Source: CAD feature listing. Evaluate the final solid. Frame: model axes, mm. A direction names the side the tool comes from. Round coordinates to 2 decimals unless told otherwise and drop trailing zeros. Order: outer loops, then holes, each group sorted by start corner. A loop starts at its lowest first (then second) coordinate and runs counter-clockwise, first axis right, second up. Notation, with made-up numbers: (6.25, -36) -> (40.25, -36) arc R19 cw to (40.25, -17) -> close; hole circle Ø9 at (86, 17.5). An arc over 180 degrees is marked (long way). Use a Markdown table: item, result. Add a question column.
Autodesk Inventor part; units mm, degrees
ref_plane "YZ Plane" through (0, 0, 0) normal (1, 0, 0) x (0, 1, 0)
ref_plane "XZ Plane" through (0, 0, 0) normal (0, 1, 0) x (-1, 0, 0)
ref_plane "XY Plane" through (0, 0, 0) normal (0, 0, 1) x (1, 0, 0)
sketch "Sketch1" plane through (0, 0, 0) normal (0, 1, 0) x (-1, 0, 0)
  line L0 (-21, 21) -> (21, 21)
  line L1 (21, 21) -> (21, -21)
  line L2 (21, -21) -> (-21, -21)
  line L3 (-21, -21) -> (-21, 21)
  line L4 (-21, 21) -> (21, -21) construction
  line L5 (21, 21) -> (-21, -21) construction
  point P0 (0, 0)
  dimension "d0" = 42
  dimension "d1" = 42
extrude "Extrusion1" add sketch "Sketch1" along normal blind 101.6
sketch "Sketch2" plane through (0, 101.6, 0) normal (0, 1, 0) x (1, 0, 0)
  line L0 (21, 21) -> (-21, 21)
  line L1 (0, 21) -> (0, 18)
  line L2 (0, 18) -> (-18, 18)
  line L3 (-18, 18) -> (18, 18)
  line L4 (18, 18) -> (18, 14)
  line L5 (18, 14) -> (-18, 14)
  line L6 (-18, 14) -> (-18, 18)
  line L7 (21, -21) -> (21, 21)
  point P0 (0, 0)
  dimension "d4" = 3
  dimension "d5" = 18
  dimension "d6" = 36
  dimension "d7" = 4
extrude "Extrusion2" cut sketch "Sketch2" against normal through all
sketch "Sketch3" plane through (21, 0, -21) normal (0, 0, -1) x (-1, 0, 0)
  line L0 (0, 101.6) -> (42, 101.6)
  line L1 (21, 101.6) -> (21, 0)
  line L2 (21, 50.8) -> (39, 50.8)
  line L3 (39, 101.6) -> (39, 0)
  circle A0 centre (21, 50.8) radius 2.125
  dimension "d10" = 4.25
extrude "Extrusion3" cut sketch "Sketch3" against normal blind 3 contours A0 L2 L1 | L1 A0 | L2 A0 L1
pattern_linear "Rectangular Pattern1" count 2 spacing 12 along (-1, 0, 0) count 4 spacing 12 along (0, 1, 0) of "Extrusion3"
pattern_linear "Rectangular Pattern2" count 4 spacing 12 along (0, 1, 0) count 2 spacing 12 along (1, 0, 0) of "Extrusion3"
sketch "Sketch4" plane through (-21, 0, -21) normal (-1, 0, 0) x (0, 0, 1)
  line L0 (42, 0) -> (42, 101.6)
  line L1 (7, 101.6) -> (7, 0)
  line L2 (7, 72.8791) -> (9, 72.8791)
  line L3 (0, 101.6) -> (42, 101.6)
  line L4 (19.3629, 101.6) -> (19.3629, 91.6)
  line L5 (21, 91.6) -> (28.5, 91.6)
  line L6 (28.5, 91.6) -> (28.5, 76.6)
  line L7 (28.5, 76.6) -> (13.5, 76.6)
  line L8 (13.5, 76.6) -> (13.5, 91.6)
  line L9 (13.5, 91.6) -> (21, 91.6)
  point P0 (21, 0)
  dimension "d25" = 2
  dimension "d26" = 10
  dimension "d27" = 91.6
  dimension "d30" = 7.5
  dimension "d31" = 15
  dimension "d32" = 15
  dimension "d33" = 15
extrude "Extrusion4" cut sketch "Sketch4" against normal through all
sketch "Sketch5" plane through (21, 0, -21) normal (0, 0, -1) x (-1, 0, 0)
  point P0 (21, 0)
sketch "Sketch6" plane through (0, 0, 0) normal (0, -1, 0) x (1, 0, 0)
  line L0 (-18, -14) -> (18, -14)
  line L1 (18, -14) -> (18, -18)
  line L2 (18, -18) -> (-18, -18)
  line L3 (-18, -18) -> (-18, -14)
  line L4 (-18, -14) -> (18, -18) construction
  line L5 (18, -14) -> (-18, -18) construction
  point P0 (0, 0)
  point P1 (0, -16)
extrude "Extrusion5" add sketch "Sketch6" against normal blind 45
sketch "Sketch7" plane through (0, 101.6, 0) normal (0, 1, 0) x (1, 0, 0)
  line L0 (-18, 18) -> (-18, -18)
  line L1 (-21, -21) -> (21, -21)
  line L2 (-18, -18) -> (18, -18)
  line L3 (18, 18) -> (18, 14)
  line L4 (18, -18) -> (18, 18)
  line L5 (18, 18) -> (-18, 18)
  point P0 (0, 0)
  dimension "d38" = 36
  dimension "d39" = 36
extrude "Extrusion6" cut sketch "Sketch7" against normal through all
sketch "Sketch8" plane through (21, 0, -21) normal (0, 0, -1) x (-1, 0, 0)
  line L0 (-0.2731, 24.5) -> (42.2731, 24.5)
  line L1 (42.2731, 24.5) -> (42.2731, -24.5)
  line L2 (42.2731, -24.5) -> (-0.2731, -24.5)
  line L3 (-0.2731, -24.5) -> (-0.2731, 24.5)
  line L4 (-0.2731, 24.5) -> (42.2731, -24.5) construction
  line L5 (42.2731, 24.5) -> (-0.2731, -24.5) construction
  point P0 (21, 0)
  dimension "d42" = 49
extrude "Extrusion7" cut sketch "Sketch8" against normal through all
sketch "Sketch9" plane through (21, 101.6, -21) normal (0, 0, -1) x (-1, 0, 0)
  circle A0 centre (33, -26.8) radius 2.125
  circle A1 centre (33, -38.8) radius 2.125
  line L0 (33, -26.8) -> (33, -38.8)
  line L1 (33, -32.8) -> (42, -32.8)
  line L2 (42, -77.1) -> (42, 0)
  line L3 (42, -32.8) -> (0, -32.8)
  line L4 (0, -32.8) -> (0, 0)
  line L5 (0, 0) -> (42, 0)
  line L6 (42, 0) -> (42, -32.8)
  circle A2 centre (21, -26.8) radius 2.125
  line L7 (21, -32.8) -> (21, -26.8)
  line L8 (42, -77.1) -> (39, -77.1)
  line L9 (0, -77.1) -> (42, -77.1)
  point P0 (21, -101.6)
  dimension "d45" = 42
  dimension "d46" = 32.8
properties part number "CraneArmBase"
1) Reachability of faces 1 (the flat face through (-20, 76.6, 0)), 2 (the cylindrical face through (-11.723, 52.907, -19.521)), 3 (the flat face through (4, 64, -18)) from +Z, -Z, +X, -X, +Y, -Y: full face, straight path, thin tool, end or side. Return the list, or none.
2) Section D-D on x = -6.5. Output: boundary loops of the cut face in (y, z).
3) Section A-A on x = -12. Output: boundary loops of the cut face in (y, z) (3 decimals).
4) Line query: probe 1 along Y at (x, z) = (-12, -19.8) (3 decimals); probe 2 along X at (y, z) = (62.8, -19) (3 decimals); probe 3 along Z at (x, y) = (9, 64.5). Output: solid intervals per line, ascending. Write a range as from..to.
5) First-contact query: pin 1 Ø6 at (y, z) = (83, 3.5) entering from +X; pin 2 Ø7 at (x, y) = (12, 74.8) entering from -Z; pin 3 Ø2.5 at (x, y) = (12, 62.8) entering from -Z. Flat tips, straight axial feed; report the tip coordinate or a pass-through.
6) Section C-C on z = -4. Output: boundary loops of the cut face in (x, y).
7) Section B-B on y = 86.8. Output: boundary loops of the cut face in (x, z) (3 decimals), then the cut area to 3 significant figures.
8) Draft query along Z for faces 4 (the cylindrical face through (0.277, 64.907, -19.521)), 5 (the flat face through (-5, 63, -21)), 6 (the flat face through (0, 63, 21)), 7 (the flat face through (-20, 84, 7.5)). Return one class per face: pulls with the +Z half, pulls with the -Z half, needs draft (parallel to the pull), parting line crosses it, or undercut.
Conclusion:
| question | item | result |
|---|---|---|
| 1 | face 1 | +X, -X |
| 1 | face 2 | -Z |
| 1 | face 3 | +Y, -Y |
| 2 | outline | (24.5, -21) -> (101.6, -21) -> (101.6, -18) -> (24.5, -18) -> close; (24.5, 18) -> (101.6, 18) -> (101.6, 21) -> (24.5, 21) -> close |
| 3 | outline | (24.5, -21) -> (48.675, -21) -> (48.675, -18) -> (24.5, -18) -> close; (24.5, 18) -> (101.6, 18) -> (101.6, 21) -> (24.5, 21) -> close; (52.925, -21) -> (60.675, -21) -> (60.675, -18) -> (52.925, -18) -> close; (64.925, -21) -> (72.675, -21) -> (72.675, -18) -> (64.925, -18) -> close; (76.925, -21) -> (84.675, -21) -> (84.675, -18) -> (76.925, -18) -> close; (88.925, -21) -> (101.6, -21) -> (101.6, -18) -> (88.925, -18) -> close |
| 4 | probe 1 | y = 24.5..48.675, 52.925..60.675, 64.925..72.675, 76.925..84.675, 88.925..101.6 |
| 4 | probe 2 | x = -21..-14.125, -9.875..-2.125, 2.125..9.875, 14.125..21 |
| 4 | probe 3 | z = -21..-18, 18..21 |
| 5 | pin 1 | passes through |
| 5 | pin 2 | stops at z = -21 |
| 5 | pin 3 | stops at z = 18 |
| 6 | outline | (-21, 24.5) -> (-18, 24.5) -> (-18, 76.6) -> (-21, 76.6) -> close; (-21, 91.6) -> (-18, 91.6) -> (-18, 101.6) -> (-21, 101.6) -> close; (18, 24.5) -> (21, 24.5) -> (21, 76.6) -> (18, 76.6) -> close; (18, 91.6) -> (21, 91.6) -> (21, 101.6) -> (18, 101.6) -> close |
| 7 | outline | (-21, -21) -> (-14.125, -21) -> (-14.125, -18) -> (-18, -18) -> (-18, -7.5) -> (-21, -7.5) -> close; (-21, 7.5) -> (-18, 7.5) -> (-18, 18) -> (18, 18) -> (18, 7.5) -> (21, 7.5) -> (21, 21) -> (-21, 21) -> close; (-9.875, -21) -> (-2.125, -21) -> (-2.125, -18) -> (-9.875, -18) -> close; (2.125, -21) -> (9.875, -21) -> (9.875, -18) -> (2.125, -18) -> close; (14.125, -21) -> (21, -21) -> (21, -7.5) -> (18, -7.5) -> (18, -18) -> (14.125, -18) -> close |
| 7 | area | 340 mm^2 |
| 8 | face 4 | needs draft |
| 8 | face 5 | pulls with the -Z half |
| 8 | face 6 | pulls with the +Z half |
| 8 | face 7 | undercut |
